Build history of the part. All positions in model axes, mm. A direction names the side the tool comes from. Give positions to 0.01 mm unless a question says otherwise; leave off trailing zeros. Write each loop counter-clockwise with the first axis right and the second up, starting at its lowest first coordinate (ties: lowest second). Pieces come first, ordered by that corner, then holes. Notation, with made-up numbers: (47, 2) -> (97, 2) arc R32 ccw to (97, 39) -> close; hole circle Ø1 at (6.25, -27.75). An arc over 180 degrees is marked (long way). Write item = value, one per line. Start each with the question number.
Q1. Tool access for faces 1 (the face through (35.4, 37.68, 1.48)), 2 (the face through (16, 38, 2)), 3 (the face through (1, 40.25, 1)): list every direction of +Z, -Z, +X, -X, +Y, -Y with a clear straight run to the whole face (end or side of a thin tool).
Q2. Wall check: line 1 (X direction, y = 6.5, z = 2); line 2 (Y direction, x = -0.5, z = 1.2); line 3 (Y direction, x = -5, z = 0.7). Give the ranges that are in metal, low to high.
Q3. Saw through at A-A, the plane y = 12.75. List the corners of the cut face in (x, z), then the cut area to 3 significant figures.
Q4. Drop flat-ended pins along their axis: P1, Ø1.5, axis at y = 34, z = 2, coming from the +X side; P2, Ø1.5, axis at y = -9.5, z = 1, coming from the -X side. Give the stop position or say it passes through.
Q5. Saw through at C-C, the plane z = 1.2. Give the number of separate pieces and of enclosed holes in the cut face, then the cut area to 3 significant figures.
Q6. Saw through at B-B, the plane x = 39. List the corners of the cut face in (y, z).
Q7. Mould opens along X. For faces 4 (the face through (40.796, 30, 2)), 5 (the face through (1.81, 22.16, 1.52)), 6 (the face through (-12.1, 39.39, 1.52)), 7 (the face through (-10, -9.75, 2)) say: pulls with the +X half, pulls with the -X half, needs draft (parallel to the pull), parting line crosses it, or undercut.
Autodesk Inventor part; units mm, degrees
ref_plane "YZ Plane" through (0, 0, 0) normal (1, 0, 0) x (0, 1, 0)
ref_plane "XZ Plane" through (0, 0, 0) normal (0, 1, 0) x (-1, 0, 0)
ref_plane "XY Plane" through (0, 0, 0) normal (0, 0, 1) x (1, 0, 0)
ref_plane "Work Plane1" through (0, 0, 0) normal (0, 0, 1) x (1, 0, 0)
sketch "Sketch1" plane through (0, 0, 0) normal (0, 0, 1) x (1, 0, 0)
  circle A0 centre (6.5, 20.75) radius 1
  circle A1 centre (6.5, 4.75) radius 1
  circle A2 centre (22.5, 20.75) radius 1
  circle A3 centre (22.5, 4.75) radius 1
  line L0 (-13, -14.75) -> (43.896, -14.75)
  line L1 (43.896, -14.75) -> (43.896, 40.25)
  line L2 (43.896, 40.25) -> (-13, 40.25)
  line L3 (-13, 40.25) -> (-13, -14.75)
  circle A4 centre (22.5, 12.75) radius 1
  circle A5 centre (14.5, 20.75) radius 1
  circle A6 centre (14.5, 4.75) radius 1
  circle A7 centre (6.5, 12.75) radius 1
  point P0 (0, 0)
  point P1 (14.5, 12.75)
  dimension "d1" = 55
  dimension "d102" = 29.396
  dimension "d103" = 27.5
  dimension "d107" = 2
  dimension "d108" = 2
  dimension "d109" = 2
  dimension "d110" = 2
extrude "Extrusion3" add sketch "Sketch1" along normal blind 3
sketch "Sketch4" plane through (0, 0, 3) normal (0, 0, 1) x (1, 0, 0)
  line L0 (42, 40.25) -> (-13, 40.25) construction
  line L1 (14.5, 40.25) -> (14.5, 12.75) construction
  line L2 (-13, 12.75) -> (14.5, 12.75) construction
  line L3 (42, 40.25) -> (-13, 40.25)
  line L4 (5, 38.2532) -> (-7, 38.25)
  line L5 (13, 40.25) -> (-7, 40.25)
  line L6 (-7, 38.25) -> (-7, 33.25)
  line L7 (-7, 33.25) -> (13, 33.25)
  line L8 (13, 40.25) -> (13, 33.25)
  line L9 (5, -7.75) -> (-13, -7.75)
  circle A0 centre (14.5, 12.75) radius 5
  line L10 (14.5, 12.75) -> (20.6229, 27.5321)
  line L11 (14.5, 12.75) -> (30.5, 12.75) construction
  circle A1 centre (20.6229, 27.5321) radius 3.895
  circle A2 centre (8.3771, 27.5321) radius 3.895
  circle A3 centre (-0.2821, 18.8729) radius 3.895
  circle A4 centre (-0.2821, 6.6271) radius 3.895
  circle A5 centre (8.3771, -2.0321) radius 3.895
  circle A6 centre (20.6229, -2.0321) radius 3.895
  circle A7 centre (29.2821, 6.6271) radius 3.895
  circle A8 centre (29.2821, 18.8729) radius 3.895
  line L12 (5, -12.75) -> (5, -7.75)
  line L13 (5, -12.75) -> (-7, -12.75)
  line L14 (-13, -7.75) -> (-13, -9.75)
  line L15 (-13, 40.25) -> (-13, -14.75)
  line L16 (-13, -9.75) -> (-7, -9.75)
  line L17 (-7, -9.75) -> (-7, -12.75)
  line L18 (-13, -14.75) -> (43.896, -14.75)
  line L19 (5, 38.2532) -> (5, 35.25)
  line L20 (5, 35.25) -> (11, 35.25)
  line L21 (11, 35.25) -> (11, 40.25)
  line L22 (24, 38.2532) -> (36, 38.25)
  line L23 (16, 40.25) -> (36, 40.25)
  line L24 (36, 38.25) -> (36, 33.25)
  line L25 (36, 33.25) -> (16, 33.25)
  line L26 (16, 40.25) -> (16, 33.25)
  line L27 (24, 38.2532) -> (24, 35.25)
  line L28 (24, 35.25) -> (18, 35.25)
  line L29 (18, 35.25) -> (18, 40.25)
  point P0 (0, 0)
  dimension "d66" = 20
  dimension "d105" = 10
  dimension "d111" = 16
  dimension "d112" = 67.5
  dimension "d113" = 7.79
  dimension "d116" = 360
  dimension "d119" = 12
  dimension "d120" = 2
  dimension "d121" = 5
  dimension "d122" = 2
  dimension "d123" = 18
  dimension "d124" = 2
  dimension "d125" = 5
  dimension "d126" = 2
  dimension "d127" = 2
  dimension "d128" = 6
  dimension "d129" = 12
  dimension "d130" = 6
extrude "Extrusion2" cut sketch "Sketch4" against normal through all
fillet "Fillet3" radius 2 14 edges at (-7, 38.25, 1.5) (5, 38.2532, 1.5) (13, 33.25, 1.5) (5, -12.75, 1.5) (-7, -12.75, 1.5) (-7, -9.75, 1.5) (-13, -9.75, 1.5) (5, 35.25, 1.5) (11, 35.25, 1.5) (16, 33.25, 1.5) (24, 35.25, 1.5) (18, 35.25, 1.5) (36, 38.25, 1.5) (24, 38.2532, 1.5)
sketch "Sketch6" plane through (0, 0, 3) normal (0, 0, 1) x (1, 0, 0)
  line L0 (43.896, 40.25) -> (-13, 40.25)
  line L1 (43.896, 40.25) -> (40.796, 40.25)
  line L2 (40.796, 40.25) -> (40.796, 20.2)
  line L3 (40.796, 20.2) -> (43.896, 20.2)
  line L4 (43.896, 20.2) -> (43.896, 40.25)
  line L5 (43.896, -14.75) -> (43.896, 40.25) construction
  line L6 (43.896, 12.75) -> (-13, 12.75) construction
  line L7 (-13, 40.25) -> (-13, -14.75) construction
  line L8 (43.896, -14.75) -> (40.796, -14.75)
  line L9 (40.796, -7.75) -> (40.796, 5.3)
  line L10 (40.796, 5.3) -> (43.896, 5.3)
  line L11 (43.896, 5.3) -> (43.896, -14.75)
  line L12 (43.896, -14.75) -> (33.896, -14.75)
  line L13 (33.896, -14.75) -> (33.896, -7.75)
  line L14 (33.896, -7.75) -> (40.796, -7.75)
  line L15 (43.896, -7.75) -> (43.896, -14.75)
  point P0 (0, 0)
  point P1 (36.3284, 40.25)
  point P2 (-13, -7.75)
  dimension "d96" = 3.1
  dimension "d97" = 20.05
  dimension "d100" = 10
  dimension "d101" = 7
extrude "Extrusion4" cut sketch "Sketch6" against normal through all
fillet "Fillet4" radius 3 1 edges at (-13, 40.25, 1.5)
equation "\"d38\" = d24"
properties part number "SideRotated"
Report:
q1.face_1 = +Z, -Z
q1.face_2 = +Z, -Z, +Y
q1.face_3 = +Z, -Z, +X, -X, +Y
q2.line_1 = -13 to -4.18, 3.61 to 25.39, 33.18 to 43.9
q2.line_2 = -14.75 to -12.75, -7.75 to 2.74, 10.52 to 14.98, 22.76 to 33.25, 38.25 to 40.25
q2.line_3 = -14.75 to -12.75, -7.75 to 33.25, 38.25 to 40.25
q3.outline = (-13, 0) -> (5.5, 0) -> (5.5, 3) -> (-13, 3) -> close; (7.5, 0) -> (9.5, 0) -> (9.5, 3) -> (7.5, 3) -> close; (19.5, 0) -> (21.5, 0) -> (21.5, 3) -> (19.5, 3) -> close; (23.5, 0) -> (43.9, 0) -> (43.9, 3) -> (23.5, 3) -> close
q3.area = 129 mm2
q4.P1 = 40.8
q4.P2 = -12.32
q5.separate_pieces = 1
q5.enclosed_holes = 17
q5.area = 2,230 mm2
q6.outline = (-7.75, 0) -> (40.25, 0) -> (40.25, 3) -> (-7.75, 3) -> close
q7.face_4 = pulls with the +X half
q7.face_5 = undercut
q7.face_6 = pulls with the -X half
q7.face_7 = needs draft
